Source: CAD feature listing. Evaluate the final solid. Frame: model axes, mm. Give positions to 0.01 mm unless a question says otherwise; leave off trailing zeros. Loops run counter-clockwise (first coordinate to the right, second up) from the corner with the lowest first, then second, coordinate; pieces in that order, holes last. Notation, with made-up numbers: M 87,2.25 L 104,2.25 A22 ccw 104,30.25 Z; hole C 15,20 d3. An arc over 180 degrees is marked long. Answer in a Markdown table with one row per item.
```python
from build123d import *

# Parameters (mm, degrees)
SKETCH_1_W      = 230
SKETCH_1_H      = 150
SKETCH_1_R      = 10
SKETCH_1_R_2    = 2.75
EXTRUDE_1_DEPTH = 5


with BuildPart() as part:
    # 草图1 → 凸台-拉伸1 (new body)
    with BuildSketch(Plane.XY):
        Rectangle(SKETCH_1_W, SKETCH_1_H)
        Circle(SKETCH_1_R, mode=Mode.SUBTRACT)
        with Locations((0, 19)):
            Circle(SKETCH_1_R_2, mode=Mode.SUBTRACT)
        with Locations((13.435028843, 13.435028843)):
            Circle(SKETCH_1_R_2, mode=Mode.SUBTRACT)
        with Locations(Location((-13.435028843, 13.435028843, 0), (0, 0, 180))):
            Circle(SKETCH_1_R_2, mode=Mode.SUBTRACT)
        with Locations(Location((13.435028843, -13.435028843, 0), (0, 0, 180))):
            Circle(SKETCH_1_R_2, mode=Mode.SUBTRACT)
        with Locations((-13.435028843, -13.435028843)):
            Circle(SKETCH_1_R_2, mode=Mode.SUBTRACT)
        with Locations(Location((0, -19, 0), (0, 0, 180))):
            Circle(SKETCH_1_R_2, mode=Mode.SUBTRACT)
        with Locations((-100, 0)):
            Circle(SKETCH_1_R_2, mode=Mode.SUBTRACT)
        with Locations((-100, 40)):
            Circle(SKETCH_1_R_2, mode=Mode.SUBTRACT)
        with Locations(Location((-100, -40, 0), (0, 0, 180))):
            Circle(SKETCH_1_R_2, mode=Mode.SUBTRACT)
        with Locations((100, -40)):
            Circle(SKETCH_1_R_2, mode=Mode.SUBTRACT)
        with Locations(Location((100, 0, 0), (0, 0, 180))):
            Circle(SKETCH_1_R_2, mode=Mode.SUBTRACT)
        with Locations(Location((100, 40, 0), (0, 0, 180))):
            Circle(SKETCH_1_R_2, mode=Mode.SUBTRACT)
    extrude(amount=EXTRUDE_1_DEPTH)


solid = part.part
```
1) Material intervals for L1, parallel to Y at x = 0, z = 3.4; L2, parallel to Y at x = -100, z = 1.6; L3, parallel to X at y = -19, z = 2.35, sorted ascending.
Reply:
| item | result |
|---|---|
| L1 | y = -75 to -21.75, -16.25 to -10, 10 to 16.25, 21.75 to 75 |
| L2 | y = -75 to -42.75, -37.25 to -2.75, 2.75 to 37.25, 42.75 to 75 |
| L3 | x = -115 to -2.75, 2.75 to 115 |
2) Section C-C, the plane y = -40. Return loops of the section in (x, z).
Reply:
| item | result |
|---|---|
| outline | M -115,0 L -102.75,0 L -102.75,5 L -115,5 Z; M -97.25,0 L 97.25,0 L 97.25,5 L -97.25,5 Z; M 102.75,0 L 115,0 L 115,5 L 102.75,5 Z |
3) Section D-D, the plane z = 3.9. Count the separate pieces of the cut face and the enclosed holes in it, then the cut area to 3 significant figures.
Reply:
| item | result |
|---|---|
| separate pieces | 1 |
| enclosed holes | 13 |
| area | 33,900 mm² |
4) Section B-B, the plane y = -19. Return loops of the section in (x, z).
Reply:
| item | result |
|---|---|
| outline | M -115,0 L -2.75,0 L -2.75,5 L -115,5 Z; M 2.75,0 L 115,0 L 115,5 L 2.75,5 Z |
5) Pull-direction query (Y, two-part tool) for faces 1 (the flat face through (115, -1, 2)), 2 (the flat face through (-2, 75, 2)), 3 (the cylindrical face through (-0.358, 21.727, 2.465)), 4 (the cylindrical face through (-97.253, -40.121, 2.465)); classes: released by +Y, released by -Y, zero draft, split by the parting line, or undercut.
Reply:
| item | result |
|---|---|
| face 1 | zero draft |
| face 2 | released by +Y |
| face 3 | undercut |
| face 4 | undercut |
6) Section A-A, the plane x = 100. Return loops of the section in (y, z), then the cut area to 4 significant figures.
Reply:
| item | result |
|---|---|
| outline | M -75,0 L -42.75,0 L -42.75,5 L -75,5 Z; M -37.25,0 L -2.75,0 L -2.75,5 L -37.25,5 Z; M 2.75,0 L 37.25,0 L 37.25,5 L 2.75,5 Z; M 42.75,0 L 75,0 L 75,5 L 42.75,5 Z |
| area | 667.5 mm² |
7) Pin query (flat end, axial travel): pin 1 Ø7 at (x, y) = (0, 19) entering from +Z. Return the tip coordinate at first contact, or that it passes through.
Reply:
| item | result |
|---|---|
| pin 1 | stops at z = 5 |
